```python
from build123d import *

# Parameters (mm, degrees)
SKETCH_1_W          = 30
SKETCH_1_H          = 70
SKETCH_1_R          = 1.6
EXTRUDE_1_DEPTH     = 3
SKETCH_2_W          = 30
SKETCH_2_H          = 3
EXTRUDE_2_DEPTH     = 32
CUT_EXTRUDE_1_REACH = 80.416
SKETCH_3_R          = 4.1
FILLET_1_R          = 3
FILLET_2_R          = 10


with BuildPart() as part:
    # 草图1 → 凸台-拉伸1 (new body)
    with BuildSketch(Plane(origin=(0, 0, 0), x_dir=(1, 0, 0), z_dir=(0, 1, 0))):
        Rectangle(SKETCH_1_W, SKETCH_1_H)
        with Locations(Location((-12, 25, 0), (0, 0, 270))):
            Circle(SKETCH_1_R, mode=Mode.SUBTRACT)
        with Locations(Location((12, 25, 0), (0, 0, 270))):
            Circle(SKETCH_1_R, mode=Mode.SUBTRACT)
        with Locations(Location((12, -2, 0), (0, 0, 270))):
            Circle(SKETCH_1_R, mode=Mode.SUBTRACT)
        with Locations(Location((-12, -2, 0), (0, 0, 270))):
            Circle(SKETCH_1_R, mode=Mode.SUBTRACT)
        with Locations(Location((10, -30, 0), (0, 0, 270))):
            Circle(SKETCH_1_R, mode=Mode.SUBTRACT)
        with Locations(Location((10, -13.8, 0), (0, 0, 270))):
            Circle(SKETCH_1_R, mode=Mode.SUBTRACT)
    extrude(amount=EXTRUDE_1_DEPTH)

    # 草图2 → 凸台-拉伸2 (add)
    with BuildSketch(Plane.XZ):
        with Locations((0, -33.5)):
            Rectangle(SKETCH_2_W, SKETCH_2_H)
    extrude(amount=EXTRUDE_2_DEPTH)

    # 草图3 → 切除-拉伸1 (cut, up to next)
    with BuildSketch(Plane(origin=(0, 0, -35), x_dir=(-1, 0, 0), z_dir=(0, 0, -1)), mode=Mode.PRIVATE) as cut_extrude_1_sk1:
        with Locations((0, -22)):
            Circle(SKETCH_3_R)
    cut_extrude_1_tool1 = extrude(cut_extrude_1_sk1.sketch, amount=-CUT_EXTRUDE_1_REACH, mode=Mode.PRIVATE) & part.part
    add(cut_extrude_1_tool1.solids().sort_by_distance((0, -22, -35))[0], mode=Mode.SUBTRACT)

    # 圆角1
    fillet_1_edges = [part.edges().sort_by_distance(p)[0] for p in [
        (15, 1.5, 35),
        (-15, 1.5, 35),
        (0, 3, -35),
    ]]
    fillet(fillet_1_edges, radius=FILLET_1_R)

    # 圆角2
    fillet_2_edges = [part.edges().sort_by_distance(p)[0] for p in [
        (15, -32, -33.5),
        (-15, -32, -33.5),
    ]]
    fillet(fillet_2_edges, radius=FILLET_2_R)


solid = part.part
```
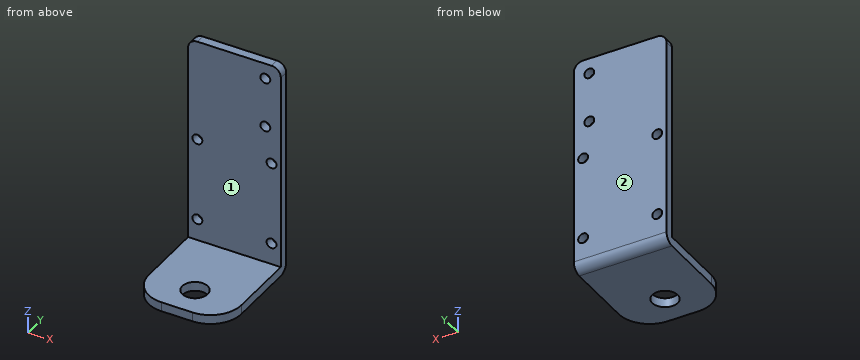
Here's how the part is built. I have some questions about the finished solid (model axes, mm). Face numbers are marked on the shaded views. A direction names the side the tool comes from. Coordinates: 2 decimals unless noted, no trailing zeros. Order: outer loops, then holes, each group sorted by start corner. A loop starts at its lowest first (then second) coordinate and runs counter-clockwise, first axis right, second up. Notation, with made-up numbers: M 27.25,60 L 34.25,60 A19 cw 34.25,94 Z; hole C -5,62.5 d9. An arc over 180 degrees is marked long. Answer as a JSON object with one key per item and string values. Group by question number.
(1) Suppose I cut it at D-D, the plane z = 13.8. Please give me the cut outline in (x, y).
(2) Suppose I cut it at A-A, the plane z = -25. Please give me the cut outline in (x, y).
(3) Which directions (+Z, -Z, +X, -X, +Y, -Y) give clear straight access to the entire face, cutting with the end or side of a thin tool? Please do the marked faces 1 and 2.
(4) For pin 1 (15 mm diameter, centred on x = 5.5, z = 12.5, fed in from -Y); pin 2 (10.5 mm diameter, centred on x = 0, y = -22, fed in from -Z); pin 3 (9 mm diameter, centred on x = 1.5, y = -17.5, fed in from +Z), each with a flat end and sliding along its axis, tell me the tip position at first contact or that it passes through.
(5) Suppose I cut it at C-C, the plane y = -23. Please give me the cut outline in (x, z).
(6) Suppose I cut it at B-B, the plane x = 0. Please give me the cut outline in (y, z).
(7) I need wall thicknesses on probe 1 along X at (y, z) = (2, 30); probe 2 along Y at (x, z) = (14, 28); probe 3 along Y at (x, z) = (0, -33.7). Which ranges of each line are inside material? Lowest first, please.
Values found:
{
 "1": {"outline": "M -15,0 L 8.4,0 L 8.4,3 L -15,3 Z; M 11.6,0 L 15,0 L 15,3 L 11.6,3 Z"},
 "2": {"outline": "M -15,0 L -13.6,0 L -13.6,3 L -15,3 Z; M -10.4,0 L 10.4,0 L 10.4,3 L -10.4,3 Z; M 13.6,0 L 15,0 L 15,3 L 13.6,3 Z"},
 "3": {"face 1": "+Z, +X, -X, -Y", "face 2": "+Z, -Z, +X, -X, +Y"},
 "4": {"pin 1": "stops at y = 0", "pin 2": "stops at z = -35", "pin 3": "stops at z = -32"},
 "5": {"outline": "M -14.95,-35 L -3.98,-35 L -3.98,-32 L -14.95,-32 Z; M 3.98,-35 L 14.95,-35 L 14.95,-32 L 3.98,-32 Z"},
 "6": {"outline": "M -32,-35 L -26.1,-35 L -26.1,-32 L -32,-32 Z; M -17.9,-35 L 0,-35 A3 ccw 3,-32 L 3,35 L 0,35 L 0,-32 L -17.9,-32 Z"},
 "7": {"probe 1": "x = -15 to 8.4, 11.6 to 15", "probe 2": "y = 0 to 3", "probe 3": "y = -32 to -26.1, -17.9 to 2.47"}
}
